```python
from build123d import *

# Parameters (mm, degrees)
BOSS_EXTRUDE1_DEPTH = 6
SKETCH2_W           = 50
SKETCH2_H           = 3
BOSS_EXTRUDE2_DEPTH = 25
CUT_EXTRUDE1_DEPTH  = 50
CUT_EXTRUDE2_DEPTH  = 25
FILLET1_R           = 5
FILLET2_R           = 2.5
CUT_EXTRUDE3_DEPTH  = 88


with BuildPart() as part:
    # Sketch1 → Boss-Extrude1 (new, symmetric)
    with BuildSketch(Plane(origin=(0, 0, 0), x_dir=(1, 0, 0), z_dir=(0, 1, 0))):
        Polygon((0, 0), (11.610474965, 0), (11.610474965, 3), (3, 3), (3, 100), (3, 103), (-47, 103), (-47, 100), (-47, 3), (-55.610474965, 3), (-55.610474965, 0), (-44, 0), (-44, 100), (0, 100), align=None)
    extrude(amount=BOSS_EXTRUDE1_DEPTH, both=True)

    # Sketch2 → Boss-Extrude2 (add, symmetric)
    with BuildSketch(Plane(origin=(0, 0, 0), x_dir=(1, 0, 0), z_dir=(0, 1, 0))):
        with Locations((-22, 101.5)):
            Rectangle(SKETCH2_W, SKETCH2_H)
    extrude(amount=BOSS_EXTRUDE2_DEPTH, both=True)

    # Sketch4 → Cut-Extrude1 (cut)
    with BuildSketch(Plane(origin=(0, 0, -3), x_dir=(-1, 0, 0), z_dir=(0, 0, -1))):
        with BuildLine():
            ThreePointArc((53.205237482, 0), (52.172824783, 1.690352707), (50.197561403, 1.543714256))
            Line((50.197561403, 1.543714256), (52.412913562, -1.543714256))
            ThreePointArc((52.412913562, -1.543714256), (52.99559019, -0.867587301), (53.205237482, 0))
        make_face()
        with BuildLine():
            Line((52.412913562, -1.543714256), (50.197561403, 1.543714256))
            ThreePointArc((50.197561403, 1.543714256), (49.761523227, -1.107676079), (52.412913562, -1.543714256))
        make_face()
    cut_extrude1 = extrude(amount=-CUT_EXTRUDE1_DEPTH, mode=Mode.SUBTRACT)

    # Mirror1: Cut-Extrude1 across plane
    add(cut_extrude1.mirror(Plane(origin=(-22, 0, 0), x_dir=(0, 0, 1), z_dir=(1, 0, 0))), mode=Mode.SUBTRACT)

    # Sketch6 → Cut-Extrude2 (cut, symmetric)
    with BuildSketch(Plane(origin=(0, 0, -103), x_dir=(-1, 0, 0), z_dir=(0, 0, -1))):
        with BuildLine():
            Line((9.5, -17.5), (34.5, -17.5))
            ThreePointArc((34.5, -17.5), (38.035533906, -16.035533906), (39.5, -12.5))
            Line((39.5, -12.5), (39.5, 12.5))
            ThreePointArc((39.5, 12.5), (38.035533906, 16.035533906), (34.5, 17.5))
            Line((34.5, 17.5), (9.5, 17.5))
            ThreePointArc((9.5, 17.5), (5.964466094, 16.035533906), (4.5, 12.5))
            Line((4.5, 12.5), (4.5, -12.5))
            ThreePointArc((4.5, -12.5), (5.964466094, -16.035533906), (9.5, -17.5))
        make_face()
    extrude(amount=CUT_EXTRUDE2_DEPTH, both=True, mode=Mode.SUBTRACT)

    # Fillet1
    fillet1_edges = [part.edges().sort_by_distance(p)[0] for p in [
        (3, 25, -101.5),
        (-47, -25, -101.5),
        (-47, 25, -101.5),
        (3, -25, -101.5),
    ]]
    fillet(fillet1_edges, radius=FILLET1_R)

    # Fillet2
    fillet2_edges = [part.edges().sort_by_distance(p)[0] for p in [
        (11.610474965, 6, -1.5),
        (-55.610474965, -6, -1.5),
        (11.610474965, -6, -1.5),
        (-44, 0, 0),
        (-47, 0, -3),
        (3, 0, -3),
        (0, 0, 0),
        (1.5, -6, -100),
        (-45.5, -6, -100),
        (-55.610474965, 6, -1.5),
        (-45.5, 6, -100),
        (1.5, 6, -100),
    ]]
    fillet(fillet2_edges, radius=FILLET2_R)

    # Sketch7 → Cut-Extrude3 (cut)
    with BuildSketch(Plane.ZY.offset(47)):
        with BuildLine():
            Line((-91.604504773, 2), (-9.5, 2))
            ThreePointArc((-9.5, 2), (-8.792893219, 1.707106781), (-8.5, 1))
            Line((-8.5, 1), (-8.5, -1))
            ThreePointArc((-8.5, -1), (-8.792893219, -1.707106781), (-9.5, -2))
            Line((-9.5, -2), (-91.604504773, -2))
            ThreePointArc((-91.604504773, -2), (-92.311611555, -1.707106781), (-92.604504773, -1))
            Line((-92.604504773, -1), (-92.604504773, 1))
            ThreePointArc((-92.604504773, 1), (-92.311611555, 1.707106781), (-91.604504773, 2))
        make_face()
    extrude(amount=-CUT_EXTRUDE3_DEPTH, mode=Mode.SUBTRACT)


solid = part.part
```
Geometry: final body of the model. Coordinates: model frame, mm. A direction names the side the tool comes from. Give positions to 0.01 mm unless a question says otherwise; leave off trailing zeros. Write each loop counter-clockwise with the first axis right and the second up, starting at its lowest first coordinate (ties: lowest second). Pieces come first, ordered by that corner, then holes.
1. Section query C-C, the plane x = -26. Return loops of the section in (y, z).
2. Section query B-B, the plane y = 10. Return loops of the section in (x, z).
3. Reachability of faces 1 (the flat face through (1, 6, -45)), 2 (the flat face through (-39.5, 0, -102)), 3 (the flat face through (10, 0, -3)) from +Z, -Z, +X, -X, +Y, -Y: full face, straight path, thin tool, end or side. Return the list, or none.
4. Draft query along X for faces 4 (the cylindrical face through (3.713, 3.334, -3.752)), 5 (the flat face through (-55.61, 0, -2)), 6 (the flat face through (-46, 0, -8.5)), 7 (the cylindrical face through (-38, -16.07, -101.52)). Return one class per face: released by +X, released by -X, zero draft, split by the parting line, or undercut.
5. Line query: probe 1 along Y at (x, z) = (1, -44); probe 2 along X at (y, z) = (-4.5, -81.5); probe 3 along Z at (x, y) = (2, 12). Output: solid intervals per line, ascending.
6. Pin query (flat end, axial travel): P1, Ø5, axis at y = -5.5, z = -76, coming from the -X side; P2, Ø1.5, axis at y = -5, z = -102, coming from the +X side; P3, Ø8, axis at y = -10.5, z = -20, coming from the +X side; P4, Ø1.8, axis at x = -53.5, y = 1.5, coming from the -Z side. Return the tip coordinate at first contact, or that it passes through.
7. Section query A-A, the plane z = -58. Return loops of the section in (x, y).
Computed:
1. outline: (-25, -103) - (-17.5, -103) - (-17.5, -100) - (-25, -100) - close; (17.5, -103) - (25, -103) - (25, -100) - (17.5, -100) - close
2. outline: (-47, -103) - (-39.5, -103) - (-39.5, -100) - (-47, -100) - close; (-4.5, -103) - (3, -103) - (3, -100) - (-4.5, -100) - close
3. face 1: +Z, +X, -X, +Y
3. face 2: +Z, -Z
3. face 3: -Z, +X, +Y, -Y
4. face 4: released by +X
4. face 5: released by -X
4. face 6: zero draft
4. face 7: undercut
5. probe 1: y = -6 to -2, 2 to 6
5. probe 2: x = -47 to -44, 0 to 3
5. probe 3: z = -103 to -100
6. P1: stops at x = -47
6. P2: stops at x = 3
6. P3: passes through
6. P4: stops at z = -3
7. outline: (-47, -6) - (-44, -6) - (-44, -2) - (-47, -2) - close; (-47, 2) - (-44, 2) - (-44, 6) - (-47, 6) - close; (0, -6) - (3, -6) - (3, -2) - (0, -2) - close; (0, 2) - (3, 2) - (3, 6) - (0, 6) - close
